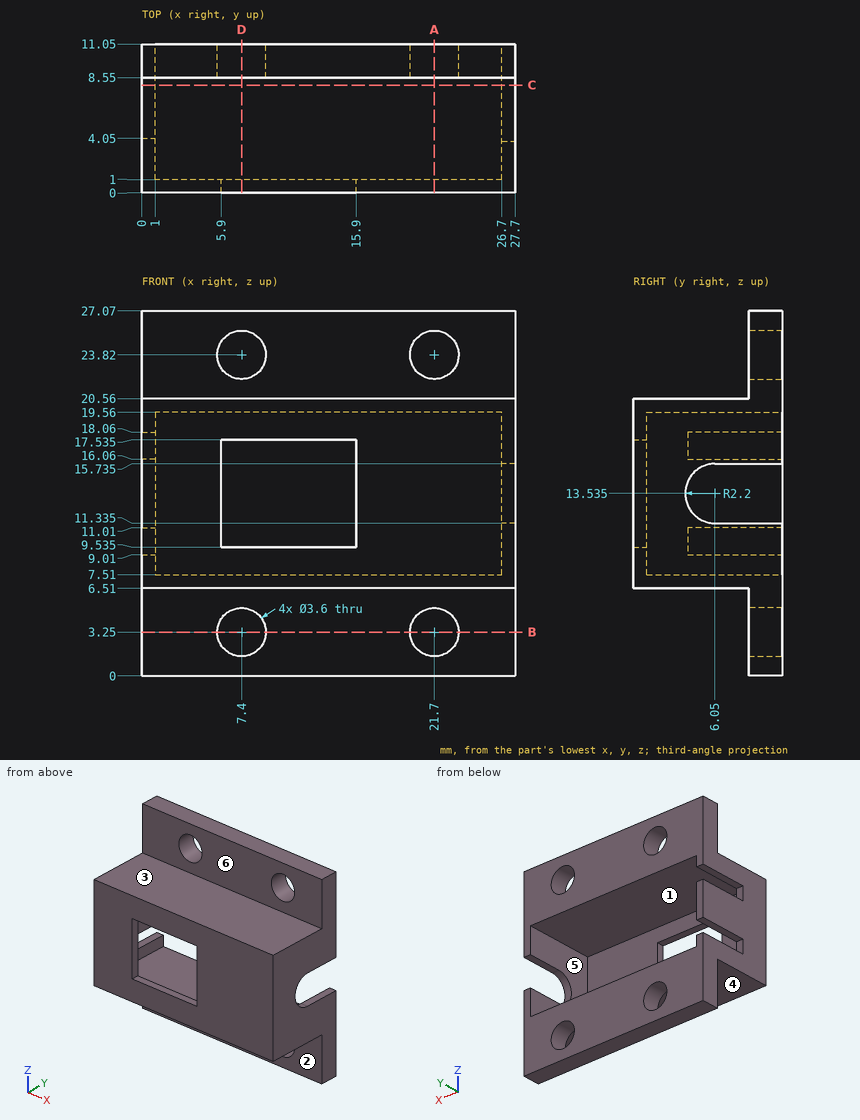
Could you check a few things on this drawing? It's one solid part, dimensions in mm from its lowest x, y, z. A direction names the side the tool comes from. Coordinates: 2 decimals unless noted, no trailing zeros. Write each loop counter-clockwise with the first axis right and the second up, starting at its lowest first coordinate (ties: lowest second). Pieces come first, ordered by that corner, then holes.
Q1. Imagine slicing it at B-B, the plane z = 3.25. List the corners of the cut face in (x, y) for me.
Results found:
outline: (0, 8.55) - (5.6, 8.55) - (5.6, 11.05) - (0, 11.05) - close; (9.2, 8.55) - (19.9, 8.55) - (19.9, 11.05) - (9.2, 11.05) - close; (23.5, 8.55) - (27.7, 8.55) - (27.7, 11.05) - (23.5, 11.05) - close
Q2. If we mould it in two halves opening along Z, with no side actions, what happens to the marked faces 4, 5 and 6? For each: +Z half, -Z half, draft (parallel to the pull), parting line (faces both ways), or undercut.
Results found:
face 4: -Z half
face 5: undercut
face 6: draft
Q3. Please list where these lines run through material, in increasing order: L1, parallel to X at y = 9.7, z = 3.25; L2, parallel to Z at x = 13.5, y = 10.5; L3, parallel to Z at x = 8, y = 9.5.
Results found:
L1: x = 0 to 5.6, 9.2 to 19.9, 23.5 to 27.7
L2: z = 0 to 7.51, 19.56 to 27.07
L3: z = 0 to 1.55, 4.95 to 7.51, 19.56 to 22.12, 25.52 to 27.07
Q4. Imagine slicing it at C-C, the plane y = 8. List the corners of the cut face in (x, z) for me (3 decimals), plus the area to 3 significant figures.
Results found:
outline: (0, 6.51) - (27.7, 6.51) - (27.7, 11.335) - (26.7, 11.335) - (26.7, 7.51) - (1, 7.51) - (1, 9.01) - (0, 9.01) - close; (0, 11.01) - (1, 11.01) - (1, 16.06) - (0, 16.06) - close; (0, 18.06) - (1, 18.06) - (1, 19.56) - (26.7, 19.56) - (26.7, 15.735) - (27.7, 15.735) - (27.7, 20.56) - (0, 20.56) - close
area: 71.1 mm2
Q5. Which directions (+Z, -Z, +X, -X, +Y, -Y) give clear straight access to the entire face, cutting with the end or side of a thin tool? Please do the marked faces 1, 2 and 3.
Results found:
face 1: +Y
face 2: -Z, +X, -X, -Y
face 3: +Z, +X, -X, -Y
Q6. Imagine slicing it at D-D, the plane x = 7.4. List the corners of the cut face in (y, z) for me (3 decimals), plus the area to 3 significant figures.
Results found:
outline: (0, 6.51) - (8.55, 6.51) - (8.55, 5.05) - (11.05, 5.05) - (11.05, 7.51) - (1, 7.51) - (1, 9.535) - (0, 9.535) - close; (0, 17.535) - (1, 17.535) - (1, 19.56) - (11.05, 19.56) - (11.05, 22.02) - (8.55, 22.02) - (8.55, 20.56) - (0, 20.56) - close; (8.55, 0) - (11.05, 0) - (11.05, 1.45) - (8.55, 1.45) - close; (8.55, 25.62) - (11.05, 25.62) - (11.05, 27.07) - (8.55, 27.07) - close
area: 40.7 mm2
Q7. For P1, Ø0.5, axis at x = 10.5, y = 0.5, coming from the +Z side; P2, Ø4, axis at x = 3.5, y = 3, coming from the -Z side; P3, Ø4, axis at x = 21.7, z = 23.82, coming from the -Y side, each with a flat end and sliding along its axis, tell me the tip position at first contact or that it passes through.
Results found:
P1: stops at z = 20.56
P2: stops at z = 6.51
P3: stops at y = 8.55
Q8. Imagine slicing it at A-A, the plane x = 21.7. List the corners of the cut face in (y, z) for me, plus the area to 3 significant figures.
Results found:
outline: (0, 6.51) - (8.55, 6.51) - (8.55, 5.05) - (11.05, 5.05) - (11.05, 7.51) - (1, 7.51) - (1, 19.56) - (11.05, 19.56) - (11.05, 22.02) - (8.55, 22.02) - (8.55, 20.56) - (0, 20.56) - close; (8.55, 0) - (11.05, 0) - (11.05, 1.45) - (8.55, 1.45) - close; (8.55, 25.62) - (11.05, 25.62) - (11.05, 27.07) - (8.55, 27.07) - close
area: 48.7 mm2
